Work out the finished part from the listing and answer in its coordinate system (mm). Round coordinates to 2 decimals unless told otherwise and drop trailing zeros. Write each loop counter-clockwise with the first axis right and the second up, starting at its lowest first coordinate (ties: lowest second). Pieces come first, ordered by that corner, then holes.
1. Find section A-A (x = 7.62). Write down the section's boundary in (y, z), and give its area (3 significant figures).
2. Find section B-B (y = 0.4). Write down the section's boundary in (x, z) (3 decimals).
3. Find section C-C (z = 0). Write down the section's boundary in (x, y) (3 decimals), and give its area (3 significant figures).
4. Find section D-D (x = -5). Write down the section's boundary in (y, z).
5. Straight lines are drawn through the part: probe 1 along X at (y, z) = (0.3, 0) (3 decimals); probe 2 along Z at (x, y) = (11.5, 0.05); probe 3 along Z at (x, y) = (14, 0.3). For each, find the intervals that lie inside material, in ascending order.
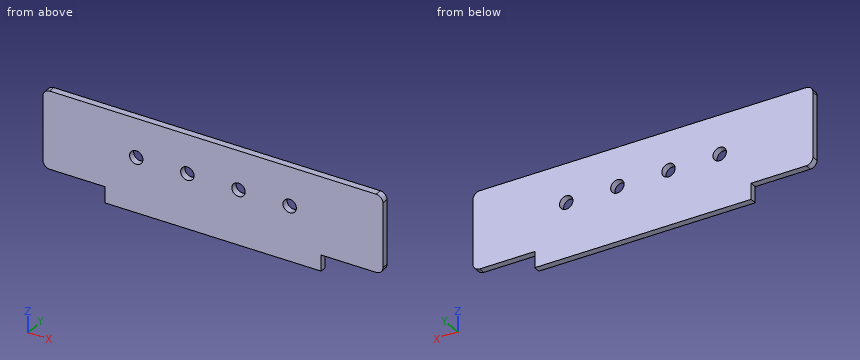
```python
from build123d import *

# Parameters (mm, degrees)
SKETCH1_R           = 0.5
BOSS_EXTRUDE1_DEPTH = 0.5


with BuildPart() as part:
    # Sketch1 → Boss-Extrude1 (new body)
    with BuildSketch(Plane(origin=(0, 0, 0), x_dir=(1, 0, 0), z_dir=(0, 1, 0))):
        with BuildLine():
            Line((13.775, 2.9), (17.875, 2.9))
            ThreePointArc((17.875, 2.9), (18.228553391, 2.753553391), (18.375, 2.4))
            Line((18.375, 2.4), (18.375, -2.4))
            ThreePointArc((18.375, -2.4), (18.228553391, -2.753553391), (17.875, -2.9))
            Line((17.875, -2.9), (-6.445, -2.9))
            ThreePointArc((-6.445, -2.9), (-6.798553391, -2.753553391), (-6.945, -2.4))
            Line((-6.945, -2.4), (-6.945, 2.4))
            ThreePointArc((-6.945, 2.4), (-6.798553391, 2.753553391), (-6.445, 2.9))
            Line((-6.445, 2.9), (-2.345, 2.9))
            Line((-2.345, 2.9), (-2.345, 4.1))
            Line((-2.345, 4.1), (13.775, 4.1))
            Line((13.775, 4.1), (13.775, 2.9))
        make_face()
        with Locations(Location((0, 0, 0), (0, 0, 270))):
            Circle(SKETCH1_R, mode=Mode.SUBTRACT)
        with Locations(Location((3.81, 0, 0), (0, 0, 270))):
            Circle(SKETCH1_R, mode=Mode.SUBTRACT)
        with Locations(Location((7.62, 0, 0), (0, 0, 270))):
            Circle(SKETCH1_R, mode=Mode.SUBTRACT)
        with Locations(Location((11.43, 0, 0), (0, 0, 270))):
            Circle(SKETCH1_R, mode=Mode.SUBTRACT)
    extrude(amount=BOSS_EXTRUDE1_DEPTH)


solid = part.part
```
Worked answers:
1. outline: (0, -4.1) - (0.5, -4.1) - (0.5, -0.5) - (0, -0.5) - close; (0, 0.5) - (0.5, 0.5) - (0.5, 2.9) - (0, 2.9) - close
1. area: 3.00 mm2
2. outline: (-6.945, -2.4) arc R0.5 ccw to (-6.445, -2.9) - (-2.345, -2.9) - (-2.345, -4.1) - (13.775, -4.1) - (13.775, -2.9) - (17.875, -2.9) arc R0.5 ccw to (18.375, -2.4) - (18.375, 2.4) arc R0.5 ccw to (17.875, 2.9) - (-6.445, 2.9) arc R0.5 ccw to (-6.945, 2.4) - close; hole circle Ø1 at (0, 0); hole circle Ø1 at (3.81, 0); hole circle Ø1 at (7.62, 0); hole circle Ø1 at (11.43, 0)
3. outline: (-6.945, 0) - (-0.5, 0) - (-0.5, 0.5) - (-6.945, 0.5) - close; (0.5, 0) - (3.31, 0) - (3.31, 0.5) - (0.5, 0.5) - close; (4.31, 0) - (7.12, 0) - (7.12, 0.5) - (4.31, 0.5) - close; (8.12, 0) - (10.93, 0) - (10.93, 0.5) - (8.12, 0.5) - close; (11.93, 0) - (18.375, 0) - (18.375, 0.5) - (11.93, 0.5) - close
3. area: 10.7 mm2
4. outline: (0, -2.9) - (0.5, -2.9) - (0.5, 2.9) - (0, 2.9) - close
5. probe 1: x = -6.945 to -0.5, 0.5 to 3.31, 4.31 to 7.12, 8.12 to 10.93, 11.93 to 18.375
5. probe 2: z = -4.1 to -0.5, 0.5 to 2.9
5. probe 3: z = -2.9 to 2.9
